from build123d import *

# Parameters (mm, degrees)
CHANFREIN1_SIZE = 0.2


with BuildPart() as part:
    # Esquisse1 → Révolution1 (revolve)
    with BuildSketch(Plane.XY, mode=Mode.PRIVATE) as r_volution1_sk:
        Polygon((-53.031441654, 0), (-53.031441654, 8), (-21.831441654, 8), (-21.831441654, 7.9), (-20.131441654, 7.9), (-20.131441654, 3), (-19.131441654, 3), (-19.131441654, 1.75), (-18.031441654, 1.75), (-18.031441654, 0.75), (-12.031441654, 0.75), (-12.031441654, 0), align=None)
    revolve(r_volution1_sk.sketch.rotate(Axis((-60.261349275, 0, 0), (1, 0, 0)), 90), axis=Axis((-60.261349275, 0, 0), (1, 0, 0)))

    # Chanfrein1
    chanfrein1_edges = [part.edges().sort_by_distance(p)[0] for p in [
        (-20.131441654, 0, -7.9),
    ]]
    chamfer(chanfrein1_edges, length=CHANFREIN1_SIZE)


solid = part.part
The model under review builds one solid part; all positions refer to its coordinate system, in mm. A direction names the side the tool comes from. Coordinates: 2 decimals unless noted, no trailing zeros. Order: outer loops, then holes, each group sorted by start corner. A loop starts at its lowest first (then second) coordinate and runs counter-clockwise, first axis right, second up. Notation, with made-up numbers: (30.25, 31) -> (66.25, 31) arc R18 cw to (66.25, 53) -> close; hole circle Ø5 at (-18, 27). An arc over 180 degrees is marked (long way). Answer in a Markdown table with one row per item.
(1) Machinability: for faces 1 (the flat face through (-18.031, 1, 0)), 2 (the flat face through (-12.031, 0, 0)), which of the approach directions +Z, -Z, +X, -X, +Y, -Y give a long, thin tool a straight path to every point of the face, cutting with its end or side? Answer none if there is none.
Answers:
| item | result |
|---|---|
| face 1 | +X |
| face 2 | +Z, -Z, +X, +Y, -Y |
(2) Consider section D-D (x = -21). Write out the cut boundary in (y, z), plus the area to 3 significant figures.
Answers:
| item | result |
|---|---|
| outline | circle Ø15.8 at (0, 0) |
| area | 196 mm² |
(3) Consider section A-A (y = 0). Write out the cut boundary in (x, z), plus the area to 3 significant figures.
Answers:
| item | result |
|---|---|
| outline | (-53.03, -8) -> (-21.83, -8) -> (-21.83, -7.9) -> (-20.33, -7.9) -> (-20.13, -7.7) -> (-20.13, -3) -> (-19.13, -3) -> (-19.13, -1.75) -> (-18.03, -1.75) -> (-18.03, -0.75) -> (-12.03, -0.75) -> (-12.03, 0.75) -> (-18.03, 0.75) -> (-18.03, 1.75) -> (-19.13, 1.75) -> (-19.13, 3) -> (-20.13, 3) -> (-20.13, 7.7) -> (-20.33, 7.9) -> (-21.83, 7.9) -> (-21.83, 8) -> (-53.03, 8) -> close |
| area | 545 mm² |
(4) Wall thickness on line 1 along X through (y, z) = (7, 0); line 2 along Y through (x, z) = (-46, 1.25); line 3 along X through (y, z) = (-6, 5.25): over which ranges is each line inside the solid? List them lowest first.
Answers:
| item | result |
|---|---|
| line 1 | -53.03 to -20.13 |
| line 2 | -7.9 to 7.9 |
| line 3 | -53.03 to -21.83 |
(5) Consider section C-C (x = -47). Write out the cut boundary in (y, z), plus the area to 3 significant figures.
Answers:
| item | result |
|---|---|
| outline | circle Ø16 at (0, 0) |
| area | 201 mm² |
(6) Insertion check: pin 1 (5 mm diameter, centred on y = -6.5, z = 1.5, fed in from +X); pin 2 (2 mm diameter, centred on x = -19.5, y = -1, fed in from +Z); pin 3 (4 mm diameter, centred on x = -29.5, y = -2.5, fed in from +Z). Each pin has a flat end and moves straight along its axis. Give the tip position at first contact, or say it passes through.
Answers:
| item | result |
|---|---|
| pin 1 | x = -20.13 |
| pin 2 | z = 7.89 |
| pin 3 | z = 7.98 |
